from build123d import *

# Parameters (mm, degrees)
BOSS_EXTRUDE1_DEPTH                                 = 12.7
CBORE_FOR_M6_HEX_SOCKET_HEAD_CAP_SCREW1_D           = 6.6
CBORE_FOR_M6_HEX_SOCKET_HEAD_CAP_SCREW1_CBORE_D     = 11
CBORE_FOR_M6_HEX_SOCKET_HEAD_CAP_SCREW1_CBORE_DEPTH = 7


with BuildPart() as part:
    # Sketch1 → Boss-Extrude1 (new, symmetric)
    with BuildSketch(Plane(origin=(0, 0, 0), x_dir=(0, 0, -1), z_dir=(1, 0, 0))):
        Polygon((0, 0), (82.446481614, 0), (82.446481614, 25.4), (65, 31.75), (0, 31.75), align=None)
    extrude(amount=BOSS_EXTRUDE1_DEPTH, both=True)

    # CBORE for M6 Hex Socket Head Cap Screw1 (through all)
    with Locations(Plane(origin=(0, 31.75, 0), x_dir=(1, 0, 0), z_dir=(0, 1, 0))):
        with Locations((0, 9.446481614), (0, 34.446481614)):
            CounterBoreHole(CBORE_FOR_M6_HEX_SOCKET_HEAD_CAP_SCREW1_D / 2, CBORE_FOR_M6_HEX_SOCKET_HEAD_CAP_SCREW1_CBORE_D / 2, CBORE_FOR_M6_HEX_SOCKET_HEAD_CAP_SCREW1_CBORE_DEPTH)


solid = part.part
The listing builds one solid part. Answer for the finished solid, in the listing's coordinates (mm). A direction names the side the tool comes from. Give positions to 0.01 mm unless a question says otherwise; leave off trailing zeros. Loops run counter-clockwise (first coordinate to the right, second up) from the corner with the lowest first, then second, coordinate; pieces in that order, holes last.
Item 1: A cutting plane is placed at D-D (z = -73.5). Give the vertices of the cut face in (x, y), then the cut area to 3 significant figures.
Derived:
outline: (-12.7, 0) - (12.7, 0) - (12.7, 28.66) - (-12.7, 28.66) - close
area: 728 mm2
Item 2: Find the intervals of material crossed by line 1 along Z through (x, y) = (0, 13.5); line 2 along Z through (x, y) = (0.75, 22.5); line 3 along X through (y, z) = (28.5, -13), in increasing order.
Derived:
line 1: z = -82.45 to -37.75, -31.15 to -12.75, -6.15 to 0
line 2: z = -82.45 to -37.66, -31.23 to -12.66, -6.23 to 0
line 3: x = -12.7 to -4.2, 4.2 to 12.7
Item 3: A cutting plane is placed at A-A (x = 0). Give the vertices of the cut face in (y, z), then the cut area to 3 significant figures.
Derived:
outline: (0, -82.45) - (25.4, -82.45) - (31.75, -65) - (31.75, -39.95) - (24.75, -39.95) - (24.75, -37.75) - (0, -37.75) - close; (0, -31.15) - (24.75, -31.15) - (24.75, -28.95) - (31.75, -28.95) - (31.75, -14.95) - (24.75, -14.95) - (24.75, -12.75) - (0, -12.75) - close; (0, -6.15) - (24.75, -6.15) - (24.75, -3.95) - (31.75, -3.95) - (31.75, 0) - (0, 0) - close
area: 2,080 mm2
Item 4: A tool of negligible diameter and unlimited length cuts with its end or side. For faces 1 (the cylindrical face through (0.43, 12.2, -12.72)), 2 (the flat face through (-0.1, 24.75, -30.9)), from which of +Z, -Z, +X, -X, +Y, -Y can it reach the whole face along a straight path? Write none if from no direction.
Derived:
face 1: +Y, -Y
face 2: +Y
Item 5: A cutting plane is placed at B-B (y = 5.5). Give the vertices of the cut face in (x, z).
Derived:
outline: (-12.7, -82.45) - (12.7, -82.45) - (12.7, 0) - (-12.7, 0) - close; hole circle Ø6.6 at (0, -34.45); hole circle Ø6.6 at (0, -9.45)
Item 6: A cutting plane is placed at C-C (x = 8.25). Give the vertices of the cut face in (y, z).
Derived:
outline: (0, -82.45) - (25.4, -82.45) - (31.75, -65) - (31.75, 0) - (0, 0) - close
Item 7: Each of these flat-tipped pins is pushed along its axis until it touches: pin 1 Ø8 at (x, y) = (-9.5, 4) entering from +Z; pin 2 Ø4 at (x, z) = (0, -34.45) entering from +Y. Where does it stop, or does it pass through?
Derived:
pin 1: stops at z = 0
pin 2: passes through
